Input: part model. Units: mm. Frame: model coordinates. A direction names the side the tool comes from. Coordinates: 2 decimals unless noted, no trailing zeros. Loops run counter-clockwise (first coordinate to the right, second up) from the corner with the lowest first, then second, coordinate; pieces in that order, holes last. Notation, with made-up numbers: (66, -4.5) -> (82, -4.5) arc R22 cw to (82, 14.5) -> close; hole circle Ø3 at (47, 25.5). An arc over 180 degrees is marked (long way). Answer as a JSON object with one key per item and string values.
from build123d import *

# Parameters (mm, degrees)
F0_W     = 5
F0_H     = 2
F1_DEPTH = 3.5
F2_SIZE  = 3
F3_R     = 1
F6_DEPTH = 9.2


with BuildPart() as f1:
    # F0 (on Top) → F1 (new body)
    with BuildSketch(Plane.XY):
        Polygon((-4.0418434781, -8.107062112), (0, -15.1077403724), (0, 7.5538701862), (-5, 7.5538701862), (-13.0836869563, 7.5538701862), (-9.0418434781, 0.5531919258), (-6.5418434781, -3.7769350931), align=None)
        Polygon((0, 7.5538701862), (0, -15.1077403724), (4.0418434781, -8.107062112), (6.5418434781, -3.7769350931), (9.0418434781, 0.5531919258), (13.0836869563, 7.5538701862), (5, 7.5538701862), align=None)
        Polygon((-10.7738942857, -0.4468080742), (-8.2738942857, -4.7769350931), (-6.5418434781, -3.7769350931), (-9.0418434781, 0.5531919258), align=None)
        Polygon((-8.2738942857, -4.7769350931), (-5.7738942857, -9.107062112), (-4.0418434781, -8.107062112), (-6.5418434781, -3.7769350931), align=None)
        Polygon((8.2738942857, -4.7769350931), (10.7738942857, -0.4468080742), (9.0418434781, 0.5531919258), (6.5418434781, -3.7769350931), align=None)
        Polygon((4.0418434781, -8.107062112), (5.7738942857, -9.107062112), (8.2738942857, -4.7769350931), (6.5418434781, -3.7769350931), align=None)
        with Locations((2.5, 8.5538701862)):
            Rectangle(F0_W, F0_H)
        with Locations((-2.5, 8.5538701862)):
            Rectangle(F0_W, F0_H)
        Polygon((-28.9386550611, -16.7077402895), (-1.3856406939, -16.7077402895), (-5.7738942857, -9.107062112), (-8.2738942857, -4.7769350931), (-10.7738942857, -0.4468080742), (-15.1621478775, 7.1538701033), align=None)
        Polygon((5.7738942857, -9.107062112), (1.3856406939, -16.7077402895), (28.9386550611, -16.7077402895), (15.1621478775, 7.1538701033), (10.7738942857, -0.4468080742), (8.2738942857, -4.7769350931), align=None)
        Polygon((5, 9.5538701862), (13.7765071836, 9.5538701862), (0, 33.415480579), (0, 9.5538701862), align=None)
        Polygon((0, 9.5538701862), (0, 33.415480579), (-13.7765071836, 9.5538701862), (-5, 9.5538701862), align=None)
    extrude(amount=F1_DEPTH)

    # F2
    f2_edges = [f1.edges().sort_by_distance(p)[0] for p in [
        (-11.062765, 4.053531, 3.5),
        (-9.907869, 0.053192, 3.5),
        (-12.968021, 3.353531, 3.5),
        (-22.050401, -4.776935, 3.5),
        (-15.162148, -16.70774, 3.5),
        (-3.579767, -12.907401, 3.5),
        (-4.907869, -8.607062, 3.5),
        (-2.020922, -11.607401, 3.5),
        (2.020922, -11.607401, 3.5),
        (4.907869, -8.607062, 3.5),
        (3.579767, -12.907401, 3.5),
        (15.162148, -16.70774, 3.5),
        (22.050401, -4.776935, 3.5),
        (12.968021, 3.353531, 3.5),
        (9.907869, 0.053192, 3.5),
        (11.062765, 4.053531, 3.5),
        (9.041843, 7.55387, 3.5),
        (5, 8.55387, 3.5),
        (9.388254, 9.55387, 3.5),
        (6.888254, 21.484675, 3.5),
        (-6.888254, 21.484675, 3.5),
        (-9.388254, 9.55387, 3.5),
        (-5, 8.55387, 3.5),
        (-9.041843, 7.55387, 3.5),
    ]]
    chamfer(f2_edges, length=F2_SIZE)

    # F3
    f3_edges = [f1.edges().sort_by_distance(p)[0] for p in [
        (-28.938655, -16.70774, 0.25),
        (28.938655, -16.70774, 0.25),
        (0, 33.415481, 0.25),
        (-15.162148, 7.15387, 0.25),
        (15.162148, 7.15387, 0.25),
        (-1.385641, -16.70774, 0.25),
        (1.385641, -16.70774, 0.25),
        (-13.083687, 7.55387, 0.25),
        (13.083687, 7.55387, 0.25),
        (0, -15.10774, 0.25),
    ]]
    fillet(f3_edges, radius=F3_R)

    # F4: F1 across plane


with BuildPart() as f1_1:
    add(f1.part)
    add(f1.part.mirror(Plane.XY))

    # F5 (on face) → F6 (cut)
    with BuildSketch(Plane.XY.offset(3.5)):
        Polygon((-2.8427077909, 20.5582287163), (2.8427077909, 20.5582287163), (0, 25.4819430411), align=None)
    extrude(amount=-F6_DEPTH, mode=Mode.SUBTRACT)


solid = f1_1.part
1. Pin query (flat end, axial travel): P1, Ø1.5, axis at y = 27.5, z = 0, coming from the +X side; P2, Ø4, axis at x = -8, z = 0.5, coming from the +Y side; P3, Ø1, axis at y = 24, z = 0, coming from the +X side; P4, Ø5, axis at x = 12, y = 0.5, coming from the +Z side. Return the tip coordinate at first contact, or that it passes through.
Reply:
{"P1": "stops at x = 3.85", "P2": "stops at y = 23.02", "P3": "stops at x = 5.72", "P4": "stops at z = 3.5"}
2. Section query C-C (x = 22.5). Return loops of the section in (y, z).
Reply:
{"outline": "(-16.71, -0.5) -> (-13.71, -3.5) -> (-11.56, -3.5) -> (-5.56, -0.5) -> (-5.56, 0.5) -> (-11.56, 3.5) -> (-13.71, 3.5) -> (-16.71, 0.5) -> close"}
3. Access query for faces 1 (the face through (-13.28, 0.85, -2.02)), 2 (the face through (-7.971, 11.075, -2.021)), 3 (the face through (-1.71, -9.11, 2.02)). Directions: +Z, -Z, +X, -X, +Y, -Y. A direction counts if a zero-diameter tool reaches every point of the face in a straight line with its end or side. Return the directions, or none.
Reply:
{"face 1": "-Z", "face 2": "-Z, -X", "face 3": "+Z"}
4. Section query D-D (z = -2.25). Return loops of the section in (x, y), plus the area to 3 significant figures.
Reply:
{"outline": "(-25.91, -14.96) -> (-4.42, -14.96) -> (-8.16, -8.47) -> (-3.4, -5.72) -> (0, -11.61) -> (3.4, -5.72) -> (8.16, -8.47) -> (4.42, -14.96) -> (25.91, -14.96) -> (15.16, 3.65) -> (11.41, -2.84) -> (6.65, -0.09) -> (10.05, 5.8) -> (3.25, 5.8) -> (3.25, 11.3) -> (10.75, 11.3) -> (0, 29.92) -> (-10.75, 11.3) -> (-3.25, 11.3) -> (-3.25, 5.8) -> (-10.05, 5.8) -> (-6.65, -0.09) -> (-11.41, -2.84) -> (-15.16, 3.65) -> close; hole (-2.84, 20.56) -> (2.84, 20.56) -> (0, 25.48) -> close", "area": "868 mm2"}
5. Section query A-A (z = 1.75). Return loops of the section in (x, y).
Reply:
{"outline": "(-26.77, -15.46) -> (-3.55, -15.46) -> (-7.48, -8.65) -> (-3.58, -6.4) -> (0, -12.61) -> (3.58, -6.4) -> (7.48, -8.65) -> (3.55, -15.46) -> (26.77, -15.46) -> (15.16, 4.65) -> (11.23, -2.15) -> (7.33, 0.1) -> (10.92, 6.3) -> (3.75, 6.3) -> (3.75, 10.8) -> (11.61, 10.8) -> (0, 30.92) -> (-11.61, 10.8) -> (-3.75, 10.8) -> (-3.75, 6.3) -> (-10.92, 6.3) -> (-7.33, 0.1) -> (-11.23, -2.15) -> (-15.16, 4.65) -> close; hole (-2.84, 20.56) -> (2.84, 20.56) -> (0, 25.48) -> close"}
6. Section query B-B (y = 8.5). Return loops of the section in (x, z).
Reply:
{"outline": "(-5, -0.5) -> (-2, -3.5) -> (2, -3.5) -> (5, -0.5) -> (5, 0.5) -> (2, 3.5) -> (-2, 3.5) -> (-5, 0.5) -> close"}
7. Mould query, pull axis X, two halves, no side actions, for faces 4 (the face through (-5.825, -12.06, 2.021)), 5 (the face through (0, 20.558, 0)), 6 (the face through (-5.694, 20.511, -2.021)), 7 (the face through (5.9, 20.2, -2)). Classes: pulls with the +X half, pulls with the -X half, needs draft (parallel to the pull), parting line crosses it, or undercut.
Reply:
{"face 4": "undercut", "face 5": "undercut", "face 6": "pulls with the -X half", "face 7": "pulls with the +X half"}
8. Line query: line 1 along X through (y, z) = (-8.5, 2); line 2 along Y through (x, z) = (10, 1.5); line 3 along X through (y, z) = (3, -0.25). Output: solid intervals per line, ascending.
Reply:
{"line 1": "x = -22.47 to -7.72, -2.08 to 2.08, 7.72 to 22.47", "line 2": "y = -15.71 to -1.15, 4.21 to 6.55, 10.55 to 14.09", "line 3": "x = -17.56 to -12.76, -10.45 to 10.45, 12.76 to 17.56"}
